Geometry check sheet. Reference: the model listing, model coordinates, mm. Give positions to 0.01 mm unless a question says otherwise; leave off trailing zeros. Loops run counter-clockwise (first coordinate to the right, second up) from the corner with the lowest first, then second, coordinate; pieces in that order, holes last. Notation, with made-up numbers: (-31.75, 40.25) -> (18.25, 40.25) arc R26 cw to (18.25, 62.25) -> close; hole circle Ø1 at (-7, 41). An arc over 180 degrees is marked (long way). Write each question's results on one line, items separated by ' | '. Start each with the question number.
1) Sectioned sample at B-B on x = 17. Record the cut outline in (y, z), then the cut area to 3 significant figures.
2) Sectioned sample at C-C on x = 4.25. Record the cut outline in (y, z), then the cut area to 3 significant figures.
3) Sectioned sample at A-A on z = -0.5. Record the cut outline in (x, y).
4) Scan lines: line 1 (Y direction, x = 12.75, z = -1); line 2 (Y direction, x = 17.5, z = -3). Record each from-to range of solid material in increasing order. Write a range as from..to.
5) Depth check by flat-ended pin: pin 1 (2 mm diameter, centred on y = 39, z = 1.5, fed in from -X). Enter the tip coordinate at first touch or a pass-through.
```python
from build123d import *

# Parameters (mm, degrees)
F1_DEPTH      = 3.8
F1_DEPTH_BACK = 3.8
F2_R          = 7.5


with BuildPart() as f1:
    # F0 (on Top) → F1 (new body, two sides)
    with BuildSketch(Plane.XY) as f1_sk:
        Polygon((0, 45), (0, 0), (10, 0), (20, 0), (20, 45), align=None)
    extrude(amount=F1_DEPTH)
    extrude(f1_sk.sketch, amount=-F1_DEPTH_BACK)

    # F2
    f2_edges = [f1.edges().sort_by_distance(p)[0] for p in [
        (20, 45, 0),
        (0, 45, 0),
    ]]
    fillet(f2_edges, radius=F2_R)


solid = f1.part
```
Result:
1) outline: (0, -3.8) -> (43.5, -3.8) -> (43.5, 3.8) -> (0, 3.8) -> close | area: 331 mm^2
2) outline: (0, -3.8) -> (44.26, -3.8) -> (44.26, 3.8) -> (0, 3.8) -> close | area: 336 mm^2
3) outline: (0, 0) -> (20, 0) -> (20, 37.5) arc R7.5 ccw to (12.5, 45) -> (7.5, 45) arc R7.5 ccw to (0, 37.5) -> close
4) line 1: 0..45 | line 2: 0..43.09
5) pin 1: x = 0.02
